Check sheet for the modelled part. Datum: model origin and axes. Units: mm. Give positions to 0.01 mm unless a question says otherwise; leave off trailing zeros. Write each loop counter-clockwise with the first axis right and the second up, starting at its lowest first coordinate (ties: lowest second). Pieces come first, ordered by that corner, then holes. Notation, with made-up numbers: M 0.25,4 L 50.25,4 A31 ccw 50.25,32 Z; hole C 55,70 d10. An arc over 180 degrees is marked long. Write item = value, one per line. Start each with the question number.
1) Sectioned sample at A-A, the plane x = -288.5. Record the cut outline in (y, z).
2) Scan lines: L1, parallel to Z at x = -326, y = -3.5; L2, parallel to Y at x = -253, z = -135.5; L3, parallel to Z at x = -517, y = -71. Record each from-to range of solid material in increasing order.
3) Gauge pin test, flat ends, axial feed: pin 1 (6 mm diameter, centred on x = -478.5, y = -30, fed in from +Z); pin 2 (1.5 mm diameter, centred on x = -109.5, y = -148.5, fed in from -Z); pin 3 (1.5 mm diameter, centred on y = -135, z = -106.5, fed in from +X); pin 4 (10 mm diameter, centred on x = -7, z = 157, fed in from -Y). Record the tip position at first contact, or that the pin passes through.
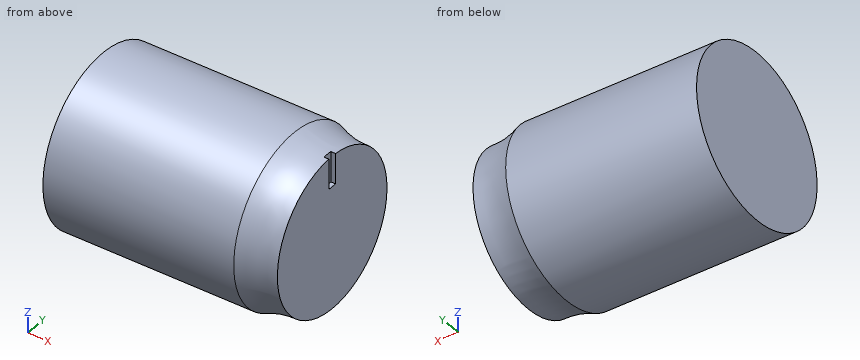
Autodesk Inventor part; units mm, degrees
ref_plane "YZ Plane" through (0, 0, 0) normal (1, 0, 0) x (0, 1, 0)
ref_plane "XZ Plane" through (0, 0, 0) normal (0, 1, 0) x (-1, 0, 0)
sketch "Sketch2" plane through (0, 0, 0) normal (0, 0, 1) x (1, 0, 0)
  line L0 (0, 0) -> (0, 200)
  arc A0 (-100, 220) -> (0, 200) centre (-6.2023, 428.9887) ccw
  line L1 (-100, 220) -> (-600, 220)
  line L2 (-600, 220) -> (-600, 0)
  line L3 (-600, 0) -> (0, 0)
  dimension "d4" = 200
  dimension "d7" = 500
revolve "Revolution1" add sketch "Sketch2" angle 360 about axis through (-600, 0, 0) along (1, 0, 0)
ref_plane "Work Plane1" through (0, 0, 120) normal (0, 0, 1) x (1, 0, 0)
sketch "Sketch3" plane through (0, 0, 120) normal (0, 0, 1) x (1, 0, 0)
  line L0 (12.5, -12.5) -> (-12.5, -12.5)
  line L1 (-12.5, -12.5) -> (-12.5, 12.5)
  line L2 (-12.5, 12.5) -> (12.5, 12.5)
  line L3 (12.5, 12.5) -> (12.5, -12.5)
  line L4 (12.5, -12.5) -> (-12.5, 12.5) construction
  line L5 (-12.5, -12.5) -> (12.5, 12.5) construction
  point P0 (0, 0)
  dimension "d10" = 25
  dimension "d11" = 25
extrude "Extrusion1" cut sketch "Sketch3" along normal blind 200
properties part number "Practica 2"
Data:
q1.outline = C 0,0 d440
q2.L1 = -219.97 to 219.97
q2.L2 = -173.32 to 173.32
q2.L3 = -208.23 to 208.23
q3.pin_1 = 218.34
q3.pin_2 = -163
q3.pin_3 = 0
q3.pin_4 = -129.86
